Autodesk Inventor part; units mm, degrees
ref_plane "YZ Plane" through (0, 0, 0) normal (1, 0, 0) x (0, 1, 0)
ref_plane "XZ Plane" through (0, 0, 0) normal (0, 1, 0) x (-1, 0, 0)
ref_plane "XY Plane" through (0, 0, 0) normal (0, 0, 1) x (1, 0, 0)
sketch "Sketch1" plane through (0, 0, 0) normal (0, 0, 1) x (1, 0, 0)
  line L0 (-22.3671, -44.8758) -> (185.479, -164.8758)
  line L1 (263.2049, -120.0008) -> (263.2049, 119.9992)
  line L2 (263.2049, 138.0318) -> (240.8188, 150.9564)
  line L3 (201.0957, -173.8921) -> (223.4817, -160.9675)
  line L4 (-37.9837, -10.0104) -> (-37.9837, -35.8596)
  line L5 (263.2049, 138.0318) -> (263.2049, -138.0333)
  line L6 (201.0957, -173.8921) -> (-37.9837, -35.8596)
  line L7 (-37.9837, 9.9896) -> (-17.9837, 9.9896)
  line L8 (-17.9837, 9.9896) -> (-17.9837, -10.0104)
  line L9 (-17.9837, -10.0104) -> (-37.9837, -10.0104)
  line L10 (-37.9837, -35.8596) -> (-37.9837, -10.0104)
  line L11 (-37.9837, 9.9896) -> (-37.9837, 35.8388)
  line L12 (223.49, -160.9627) -> (213.49, -143.6422)
  line L13 (213.49, -143.6422) -> (230.8105, -133.6422)
  line L14 (230.8105, -133.6422) -> (240.8105, -150.9627)
  line L15 (263.2049, -138.0333) -> (240.8105, -150.9627)
  line L16 (223.49, -160.9627) -> (201.0957, -173.8921)
  line L17 (223.5235, 160.9901) -> (213.4873, 143.6905)
  line L18 (213.4873, 143.6905) -> (230.7869, 133.6543)
  line L19 (230.7869, 133.6543) -> (240.7869, 150.9748)
  line L20 (201.1375, 173.9147) -> (223.5235, 160.9901)
  line L21 (240.7869, 150.9748) -> (263.2049, 138.0318)
  line L22 (-37.9837, 35.8388) -> (201.1375, 173.9147)
  point P0 (0, 0)
  dimension "d0" = 20
  dimension "d1" = 20
  dimension "d2" = 20
  dimension "d3" = 20
  dimension "d4" = 20
  dimension "d5" = 20
extrude "Extrusion1" add sketch "Sketch1" along normal blind 6.35
sketch "Sketch2" plane through (0, 0, 6.35) normal (0, 0, 1) x (1, 0, 0)
  line L0 (201.1375, 173.9147) -> (-37.9837, 35.8388)
  line L1 (-37.9837, -35.8596) -> (201.0957, -173.8921)
  line L2 (263.2049, -138.0333) -> (263.2049, 138.0318)
  line L3 (-13.2714, -20.105) -> (-13.2714, 20.0856)
  line L4 (237.2204, -124.5359) -> (202.4143, -144.6312)
  line L5 (202.4143, 144.6118) -> (237.2204, 124.5165)
  line L6 (-13.2714, -0.0097) -> (263.2049, -0.0008) construction
  line L7 (219.8173, 134.5641) -> (81.556, -104.8758) construction
  line L8 (219.8173, -134.5836) -> (81.5535, 104.8633) construction
  circle A0 centre (142.1099, -0.009) radius 90 construction
  line L9 (-13.2714, -21.259) -> (29.2286, -21.259) construction
  line L10 (29.2286, -21.259) -> (29.2286, 21.241) construction
  line L11 (29.2286, 21.241) -> (-13.2714, 21.241) construction
  line L12 (-13.2714, 21.241) -> (-13.2714, -21.259) construction
  line L13 (-13.2714, -21.259) -> (29.2286, 21.241) construction
  line L14 (29.2286, -21.259) -> (-13.2714, 21.241) construction
  line L15 (-7.5214, -15.509) -> (23.4786, -15.509) construction
  line L16 (23.4786, -15.509) -> (23.4786, 15.491) construction
  line L17 (23.4786, 15.491) -> (-7.5214, 15.491) construction
  line L18 (-7.5214, 15.491) -> (-7.5214, -15.509) construction
  line L19 (-7.5214, -15.509) -> (23.4786, 15.491) construction
  line L20 (23.4786, -15.509) -> (-7.5214, 15.491) construction
  point P0 (0, 0)
  point P1 (7.9786, -0.009)
  point P2 (203.5022, -137.3435)
  point P3 (188.0022, -110.4967)
  point P4 (214.849, -94.9967)
  point P5 (230.349, -121.8435)
  point P6 (230.3489, 121.8255)
  point P7 (214.8489, 94.9787)
  point P8 (188.0021, 110.4787)
  point P9 (203.5021, 137.3255)
  dimension "d8" = 180
  dimension "d9" = 42.5
  dimension "d10" = 42.5
  dimension "d11" = 31
  dimension "d12" = 31
  dimension "d15" = 360
hole "Hole1" at (-7.5214, 15.491, 6.35) at (23.4786, 15.491, 6.35) at (23.4786, -15.509, 6.35) at (-7.5214, -15.509, 6.35) at (230.349, -121.8435, 6.35) at (214.849, -94.9967, 6.35) at (188.0022, -110.4967, 6.35) at (203.5022, -137.3435, 6.35) at (203.5021, 137.3255, 6.35) at (188.0021, 110.4787, 6.35) at (214.8489, 94.9787, 6.35) at (230.3489, 121.8255, 6.35) direction (0, 0, -1) diameter 3.4 end through all
sketch "Sketch3" plane through (0, 0, 6.35) normal (0, 0, 1) x (1, 0, 0)
  circle A0 centre (23.4786, -15.509) radius 1.7
  circle A1 centre (-7.5214, 15.491) radius 1.7
  line L0 (-17.9837, 9.9896) -> (-17.9837, -10.0104)
  line L1 (213.49, -143.6422) -> (230.8105, -133.6422)
  line L2 (230.7869, 133.6543) -> (213.4873, 143.6905)
  line L3 (-7.5214, 15.491) -> (23.4786, -15.509) construction
  circle A2 centre (7.9786, -0.009) radius 11.25
  circle A3 centre (142.1124, 0.0111) radius 160.0962 construction
  circle A4 centre (209.1968, -116.1422) radius 11.25
  circle A5 centre (209.1619, 116.1844) radius 11.25
  point P0 (0, 0)
  dimension "d24" = 22.5
  dimension "d27" = 360
extrude "Extrusion2" cut sketch "Sketch3" against normal through all contours A2 | A4 | A5
sketch "Sketch4" plane through (0, 0, 6.35) normal (0, 0, 1) x (1, 0, 0)
  line L0 (201.1375, 173.9147) -> (-37.9837, 35.8388)
  line L1 (-37.9837, -35.8596) -> (201.0957, -173.8921)
  line L2 (263.2049, -138.0333) -> (263.2049, 138.0318)
  circle A0 centre (-13.6913, -49.8848) radius 10 construction
  circle A1 centre (176.8343, -159.8848) radius 10 construction
  line L3 (-8.6913, -41.2245) -> (181.8343, -151.2245) construction
  line L4 (-22.3516, -44.8848) -> (-12.3516, -27.5643) construction
  line L5 (195.4945, -147.5643) -> (185.4945, -164.8848) construction
  circle A2 centre (142.1084, -0.0056) radius 121.0965 construction
  point P0 (0, 0)
  point P1 (86.5715, -96.2245)
  point P2 (253.2049, 0.0075)
  point P3 (253.2049, -109.9925)
  point P4 (253.2049, 110.0075)
  point P5 (86.5488, 96.2003)
  point P6 (181.8115, 151.2003)
  point P7 (-8.714, 41.2003)
  dimension "d31" = 20
  dimension "d32" = 20
  dimension "d35" = 360
hole "Hole2" at (86.5715, -96.2245, 6.35) at (-8.6913, -41.2245, 6.35) at (181.8343, -151.2245, 6.35) at (253.2049, -109.9925, 6.35) at (253.2049, 0.0075, 6.35) at (253.2049, 110.0075, 6.35) at (181.8115, 151.2003, 6.35) at (86.5488, 96.2003, 6.35) at (-8.714, 41.2003, 6.35) direction (0, 0, -1) diameter 4.5 end through all
sketch "Sketch5" plane through (0, 0, 6.35) normal (0, 0, 1) x (1, 0, 0)
  line L0 (201.1375, 173.9147) -> (-37.9837, 35.8388)
  line L1 (-37.9837, -35.8596) -> (201.0957, -173.8921)
  line L2 (263.2049, -138.0333) -> (263.2049, 138.0318)
  circle A0 centre (142.1084, -0.0056) radius 121.0965 construction
  circle A1 centre (142.1084, -0.0056) radius 95 construction
  circle A2 centre (47.0693, 0.6182) radius 12.5 construction
  arc A3 (71.6251, 63.6899) -> (52.1084, 30.4082) centre (142.1084, -0.0056) ccw construction
  arc A4 (67.9155, 67.0423) -> (47.3715, 32.009) centre (142.1084, -0.0056) ccw
  arc A5 (75.3347, 60.3375) -> (56.8452, 28.8075) centre (142.1084, -0.0056) ccw
  arc A6 (75.3347, 60.3375) -> (67.9155, 67.0423) centre (71.6251, 63.6899) ccw
  arc A7 (47.3715, 32.009) -> (56.8452, 28.8075) centre (52.1084, 30.4082) ccw
  circle A8 centre (47.0693, 0.6182) radius 5
  circle A9 centre (94.0486, -81.9999) radius 5
  circle A10 centre (189.0877, -82.6237) radius 5
  circle A11 centre (237.1474, -0.6294) radius 5
  circle A12 centre (190.1681, 81.9888) radius 5
  circle A13 centre (95.129, 82.6126) radius 5
  point P0 (0, 0)
  point P1 (48.0142, 13.0824)
  point P2 (47.8506, -11.8574)
  point P3 (83.7268, -74.9495)
  point P4 (105.2434, -87.5611)
  point P5 (177.8209, -88.0375)
  point P6 (199.5012, -75.7093)
  point P7 (236.2025, -13.0936)
  point P8 (236.3662, 11.8462)
  point P9 (200.49, 74.9383)
  point P10 (178.9733, 87.55)
  point P11 (106.3959, 88.0263)
  point P12 (84.7155, 75.6982)
  dimension "d45" = 190
  dimension "d46" = 25
  dimension "d49" = 360
  dimension "d60" = 10
  dimension "d63" = 360
extrude "Extrusion3" cut sketch "Sketch5" against normal through all contours A6 A5 A7 A4
hole "Hole3" at (48.0142, 13.0824, 6.35) at (47.8506, -11.8574, 6.35) at (83.7268, -74.9495, 6.35) at (105.2434, -87.5611, 6.35) at (177.8209, -88.0375, 6.35) at (199.5012, -75.7093, 6.35) at (236.2025, -13.0936, 6.35) at (236.3662, 11.8462, 6.35) at (200.49, 74.9383, 6.35) at (178.9733, 87.55, 6.35) at (106.3959, 88.0263, 6.35) at (84.7155, 75.6982, 6.35) direction (0, 0, -1) diameter 3.4 end through all
extrude "Extrusion4" cut sketch "Sketch5" against normal through all contours A8 | A9 | A10 | A11 | A12 | A13
properties part number "build deck"
Design review of the part built by this model. Coordinates are the model's own, in mm. A direction names the side the tool comes from. Coordinates: 2 decimals unless noted, no trailing zeros. Order: outer loops, then holes, each group sorted by start corner. A loop starts at its lowest first (then second) coordinate and runs counter-clockwise, first axis right, second up. Notation, with made-up numbers: M -5.75,-10.5 L 41.25,-10.5 A19 cw 41.25,26.5 Z; hole C 8.5,63.5 d3. An arc over 180 degrees is marked long. Use a Markdown table: item, result.
(1) Draft analysis for pull direction Y (two halves, no side actions). For faces 1 (the flat face through (235.717, 142.193, 3.131)), 2 (the flat face through (235.74, -142.18, 3.13)), 3 (the cylindrical face through (194.937, 83.491, 3.219)), state which applies: released by +Y, released by -Y, zero draft, split by the parting line, or undercut.
Worked answers:
| item | result |
|---|---|
| face 1 | released by +Y |
| face 2 | released by -Y |
| face 3 | undercut |
(2) For faces 4 (the cylindrical face through (64.6, 45.74, 3.22)), 5 (the flat face through (144, 2, 0)), list the 3-axis set-ups (+Z, -Z, +X, -X, +Y, -Y) from which the entire face can be reached by the end or side of a thin tool; tool diameter is ignored.
Worked answers:
| item | result |
|---|---|
| face 4 | +Z, -Z |
| face 5 | -Z, +X, -X, +Y, -Y |
(3) Wall thickness on probe 1 along Y at (x, z) = (211, 1.5); probe 2 along X at (y, z) = (0.5, 2.25); probe 3 along X at (y, z) = (137, 1.5): over which ranges is each line inside the solid? List them lowest first.
Worked answers:
| item | result |
|---|---|
| probe 1 | y = -168.17 to -127.25, -105.04 to 105.09, 127.28 to 168.22 |
| probe 2 | x = -17.98 to -3.26, 19.22 to 42.07, 52.07 to 232.28, 242.02 to 251.01, 255.4 to 263.2 |
| probe 3 | x = 137.21 to 201.83, 205.17 to 225.02, 232.72 to 263.2 |
(4) Add section B-B (x = 121). Give the boundary of the cut face in (y, z), then the cut area to 3 significant figures.
Worked answers:
| item | result |
|---|---|
| outline | M -127.65,0 L 127.64,0 L 127.64,6.35 L -127.65,6.35 Z |
| area | 1,620 mm2 |
(5) Add section A-A (z = 2.75). Count the separate pieces of the cut face and the enclosed holes in it, then the cut area to 3 significant figures.
Worked answers:
| item | result |
|---|---|
| separate pieces | 1 |
| enclosed holes | 43 |
| area | 65,800 mm2 |
(6) For P1, Ø3.5, axis at x = 253.2, y = 0.01, coming from the +Z side; P2, Ø2, axis at x = -7.5, z = 4, coming from the +Y side, all flat-tipped, find the tip position at first contact; note any pin that passes through.
Worked answers:
| item | result |
|---|---|
| P1 | passes through |
| P2 | stops at y = 54.02 |
